```python
from build123d import *

# Parameters (mm, degrees)
MODEL_R                 = 2.4
MODEL_R_2               = 2
SALIENTE_EXTRUIR1_DEPTH = 3


with BuildPart() as part:
    # Model → Saliente-Extruir1 (new body)
    with BuildSketch(Plane.XY):
        with BuildLine():
            Line((60.128031424, 43.810084434), (60.128031424, 26.988429812))
            Line((60.128031424, 26.988429812), (60.128031424, 8.810084434))
            ThreePointArc((60.128031424, 8.810084434), (61.592497518, 5.274550528), (65.128031424, 3.810084434))
            Line((65.128031424, 3.810084434), (103.128031424, 3.810084434))
            ThreePointArc((103.128031424, 3.810084434), (106.66356533, 5.274550528), (108.128031424, 8.810084434))
            Line((108.128031424, 8.810084434), (108.128031424, 43.810084434))
            Line((108.128031424, 43.810084434), (97.128031424, 43.810084434))
            Line((97.128031424, 43.810084434), (97.128031424, 33.810084434))
            Line((97.128031424, 33.810084434), (100.128031424, 33.810084434))
            Line((100.128031424, 33.810084434), (100.128031424, 30.810084434))
            Line((100.128031424, 30.810084434), (90.128031424, 30.810084434))
            Line((90.128031424, 30.810084434), (90.128031424, 33.810084434))
            Line((90.128031424, 33.810084434), (78.128031424, 33.810084434))
            Line((78.128031424, 33.810084434), (78.128031424, 30.810084434))
            Line((78.128031424, 30.810084434), (68.128031424, 30.810084434))
            Line((68.128031424, 30.810084434), (68.128031424, 33.810084434))
            Line((68.128031424, 33.810084434), (71.128031424, 33.810084434))
            Line((71.128031424, 33.810084434), (71.128031424, 43.810084434))
            Line((71.128031424, 43.810084434), (60.128031424, 43.810084434))
        make_face()
        with Locations((97.386085589, 13.789032772)):
            Circle(MODEL_R, mode=Mode.SUBTRACT)
        with Locations((65.128031424, 37.810084434)):
            Circle(MODEL_R_2, mode=Mode.SUBTRACT)
        with Locations((103.128031424, 37.810084434)):
            Circle(MODEL_R_2, mode=Mode.SUBTRACT)
        with BuildLine():
            Line((78.683481489, 11.277984768), (77.72633505, 11.277984768))
            ThreePointArc((77.72633505, 11.277984768), (66.483480743, 13.783830387), (77.728934453, 16.277984768))
            Line((77.728934453, 16.277984768), (78.683481489, 16.277984768))
            ThreePointArc((78.683481489, 16.277984768), (81.183481489, 13.777984768), (78.683481489, 11.277984768))
        make_face(mode=Mode.SUBTRACT)
    extrude(amount=SALIENTE_EXTRUIR1_DEPTH)


solid = part.part
```
Input: part model. Units: mm. Frame: model coordinates. A direction names the side the tool comes from. Give positions to 0.01 mm unless a question says otherwise; leave off trailing zeros. Order: outer loops, then holes, each group sorted by start corner. A loop starts at its lowest first (then second) coordinate and runs counter-clockwise, first axis right, second up. Notation, with made-up numbers: (18.5, -32.75) - (61.5, -32.75) arc R35 cw to (61.5, 1.25) - close; hole circle Ø10 at (84, -0.5). An arc over 180 degrees is marked (long way). One line per item, written item: value.
1. Cut plane C-C, the plane z = 1.3. Output: boundary loops of the cut face in (x, y), and give its area (3 significant figures).
Determined:
outline: (60.13, 8.81) arc R5 ccw to (65.13, 3.81) - (103.13, 3.81) arc R5 ccw to (108.13, 8.81) - (108.13, 43.81) - (97.13, 43.81) - (97.13, 33.81) - (100.13, 33.81) - (100.13, 30.81) - (90.13, 30.81) - (90.13, 33.81) - (78.13, 33.81) - (78.13, 30.81) - (68.13, 30.81) - (68.13, 33.81) - (71.13, 33.81) - (71.13, 43.81) - (60.13, 43.81) - close; hole circle Ø4 at (65.13, 37.81); hole (77.73, 11.28) - (78.68, 11.28) arc R2.5 ccw to (78.68, 16.28) - (77.73, 16.28) arc R5.9 ccw (long way) to start; hole circle Ø4.8 at (97.39, 13.79); hole circle Ø4 at (103.13, 37.81)
area: 1,420 mm2
2. Cut plane B-B, the plane y = 41.5. Output: boundary loops of the cut face in (x, z).
Determined:
outline: (60.13, 0) - (71.13, 0) - (71.13, 3) - (60.13, 3) - close; (97.13, 0) - (108.13, 0) - (108.13, 3) - (97.13, 3) - close
3. Pin query (flat end, axial travel): pin 1 Ø1.5 at (x, z) = (73, 2) entering from +Y; pin 2 Ø8 at (x, y) = (78, 39) entering from +Z; pin 3 Ø1.5 at (x, z) = (87, 1) entering from +Y. Return the tip coordinate at first contact, or that it passes through.
Determined:
pin 1: y = 30.81
pin 2: through
pin 3: y = 33.81
4. Reachability of faces 1 (the face through (66, 43.81, 1)), 2 (the face through (81.183, 13.833, 1.479)), 3 (the face through (78.128, 32, 1)) from +Z, -Z, +X, -X, +Y, -Y: full face, straight path, thin tool, end or side. Return the list, or none.
Determined:
face 1: +Z, -Z, +X, -X, +Y
face 2: +Z, -Z
face 3: +Z, -Z, +Y
5. Line query: probe 1 along X at (y, z) = (33, 0.15); probe 2 along Y at (x, z) = (103, 1.7); probe 3 along X at (y, z) = (41.5, 1.65). Output: solid intervals per line, ascending.
Determined:
probe 1: 60.13 to 68.13, 78.13 to 90.13, 100.13 to 108.13
probe 2: 3.81 to 35.81, 39.81 to 43.81
probe 3: 60.13 to 71.13, 97.13 to 108.13
6. Cut plane A-A, the plane y = 32.5. Output: boundary loops of the cut face in (x, z).
Determined:
outline: (60.13, 0) - (68.13, 0) - (68.13, 3) - (60.13, 3) - close; (78.13, 0) - (90.13, 0) - (90.13, 3) - (78.13, 3) - close; (100.13, 0) - (108.13, 0) - (108.13, 3) - (100.13, 3) - close
7. Cut plane D-D, the plane x = 70. Output: boundary loops of the cut face in (y, z), and give its area (3 significant figures).
Determined:
outline: (3.81, 0) - (8.38, 0) - (8.38, 3) - (3.81, 3) - close; (19.18, 0) - (30.81, 0) - (30.81, 3) - (19.18, 3) - close; (33.81, 0) - (43.81, 0) - (43.81, 3) - (33.81, 3) - close
area: 78.6 mm2
